Input: part model. Units: mm. Frame: model coordinates. A direction names the side the tool comes from. Give positions to 0.01 mm unless a question says otherwise; leave off trailing zeros. Write each loop counter-clockwise with the first axis right and the second up, starting at its lowest first coordinate (ties: lowest second). Pieces come first, ordered by that corner, then holes. Notation, with made-up numbers: (70, 74) -> (79, 74) arc R8 ccw to (79, 79) -> close; hole circle Ø9 at (-24, -7.5). An arc over 180 degrees is marked (long way). Return JSON: item names as keys, results as strings. Group by question number.
Item 1: Set-up query: faces 1 (the face through (143, 2, -49)), 2 (the face through (314.8, 0.99, -81.27)), 3 (the face through (163, 49, 0)), 4 (the face through (266.02, 0.99, -35.32)), 5 (the face through (143, 0, -51)). Return all of +Z, -Z, +X, -X, +Y, -Y with unobstructed straight access to the full face (end or side cutting, diameter ignored); none if empty.
Item 2: Section A-A, the plane y = 22. Return loops of the section in (x, z), then the cut area to 3 significant figures.
Item 3: Line query: line 1 (Z direction, x = 187, y = 1); line 2 (Z direction, x = -9, y = 61.5); line 3 (Y direction, x = 212.5, z = -59). Output: solid intervals per line, ascending. Write a range as [from, to].
Item 4: Pin query (flat end, axial travel): P1, Ø1.6, axis at y = 0.5, z = -47.5, coming from the +X side; P2, Ø5, axis at x = 196.5, y = 19, coming from the +Z side. Return the tip coordinate at first contact, or that it passes through.
Item 5: Mould query, pull axis X, two halves, no side actions, for faces 6 (the face through (266.84, 0.99, -66.93)), 7 (the face through (-50, 72.5, -98.4)), 8 (the face through (178, 98, -51)), 9 (the face through (340.31, 53.78, -0.99)). Classes: released by +X, released by -X, zero draft, split by the parting line, or undercut.
Item 6: Section D-D, the plane x = 93. Return loops of the section in (y, z), then the cut area to 3 significant figures.
Item 7: Section C-C, the plane z = -25. Return loops of the section in (x, y), then the cut area to 3 significant figures.
Item 8: Section B-B, the plane x = 151.5. Return loops of the section in (y, z).
Autodesk Inventor part; units mm, degrees
ref_plane "YZ Plane" through (0, 0, 0) normal (1, 0, 0) x (0, 1, 0)
ref_plane "XZ Plane" through (0, 0, 0) normal (0, 1, 0) x (-1, 0, 0)
ref_plane "XY Plane" through (0, 0, 0) normal (0, 0, 1) x (1, 0, 0)
sketch "Náčrt1" plane through (0, 0, 0) normal (1, 0, 0) x (0, 1, 0)
  line L0 (0, 0) -> (100, 0)
  line L1 (100, 0) -> (100, -100)
  line L2 (100, -100) -> (0, -100)
  line L3 (0, -100) -> (0, 0)
  line L4 (98, -2) -> (2, -2)
  line L5 (2, -2) -> (2, -98)
  line L6 (2, -98) -> (98, -98)
  line L7 (98, -98) -> (98, -2)
  dimension "d0" = 100
  dimension "d1" = 100
  dimension "d2" = 2
extrude "Vysunutí1" add sketch "Náčrt1" along normal blind 370
sketch "Náčrt4" plane through (0, 0, 0) normal (0, 0, 1) x (1, 0, 0)
  line L0 (0, 0) -> (0, 100)
  line L1 (0, 0) -> (370, 0)
  line L2 (370, 100) -> (370, 0)
  line L3 (0, 100) -> (370, 100)
  line L4 (0, 2) -> (370, 2)
  arc A0 (370, 98) -> (330.0148, 0) centre (465.2, 2) ccw
  line L5 (330, 23.5767) -> (330, -17.4459)
  line L6 (370, 2) -> (523.9799, 2)
  line L7 (330, 2) -> (370, 2)
  line L8 (0, 0) -> (370, 0)
  line L9 (370, 2) -> (370, 98)
  dimension "d17" = 2
  dimension "d102" = 330
extrude "Vysunutí4" cut sketch "Náčrt4" against normal through all contours A0 L2 L4 | L4 L2 L1 A0
sketch "Náčrt5" plane through (0, 100, 0) normal (0, 1, 0) x (1, 0, 0)
  line L0 (0, 0) -> (0, 100)
  line L1 (0, 0) -> (370, 0)
  line L2 (370, 100) -> (370, 0)
  line L3 (0, 100) -> (370, 100)
  arc A0 (370, 0) -> (370, 100) centre (343.3333, 50) ccw
  point P0 (400, 50)
  dimension "d21" = 30
extrude "Vysunutí5" add sketch "Náčrt5" against normal blind 2 contours L2 A0
sketch "Náčrt11" plane through (0, 0, -100) normal (0, -1, 0) x (1, 0, 0)
  line L0 (0, 100) -> (330.0148, 100)
  line L1 (0, 0) -> (0, 100)
  line L2 (0, 0) -> (330.0148, 0)
  line L3 (330.0148, 0) -> (330.0148, 100)
  line L4 (86.35, 55.65) -> (97.65, 55.65)
  line L5 (97.65, 55.65) -> (97.65, 44.35)
  line L6 (97.65, 44.35) -> (86.35, 44.35)
  line L7 (86.35, 44.35) -> (86.35, 55.65)
  point P0 (92, 55.65)
  point P1 (86.35, 50)
  dimension "d129" = 11.3
  dimension "d130" = 11.3
  dimension "d131" = 92
  dimension "d132" = 50
extrude "Vysunutí11" cut sketch "Náčrt11" against normal blind 5 contours L4 L5 L6 L7
sketch "Náčrt12" plane through (0, 0, -100) normal (0, -1, 0) x (1, 0, 0)
  line L0 (0, 100) -> (330.0148, 100)
  line L1 (0, 0) -> (0, 100)
  line L2 (0, 0) -> (330.0148, 0)
  circle A0 centre (187, 90) radius 2.25
  circle A1 centre (187, 10) radius 2.25
  line L3 (330.0148, 0) -> (330.0148, 100)
  dimension "d61" = 4.5
  dimension "d62" = 4.5
  dimension "d63" = 10
  dimension "d64" = 10
  dimension "d65" = 187
  dimension "d66" = 187
extrude "Vysunutí12" cut sketch "Náčrt12" against normal blind 10 contours A0 | A1
sketch "Náčrt14" plane through (0, 0, -100) normal (0, 0, -1) x (-1, 0, 0)
  line L0 (0, 0) -> (-330.0148, 0)
  line L1 (0, 100) -> (0, 0)
  line L2 (0, 100) -> (-370, 100)
  line L3 (-370, 98) -> (-370, 100)
  circle A0 centre (-293, 7.5) radius 2.25
  circle A1 centre (-293, 92.5) radius 2.25
  arc A2 (-330.0148, 0) -> (-370, 98) centre (-465.2, 2) ccw
  dimension "d77" = 293
  dimension "d78" = 4.5
  dimension "d79" = 4.5
  dimension "d80" = 293
  dimension "d86" = 85
  dimension "d87" = 7.5
extrude "Vysunutí14" cut sketch "Náčrt14" against normal through all contours A0 | A1
sketch "Náčrt16" plane through (0, 0, -100) normal (0, -1, 0) x (1, 0, 0)
  circle A0 centre (187, 90) radius 2.25
  circle A1 centre (187, 10) radius 2.25
  line L0 (330.0148, 0) -> (330.0148, 100)
  line L1 (0, 100) -> (330.0148, 100)
  line L2 (0, 0) -> (0, 100)
  line L3 (0, 0) -> (330.0148, 0)
  line L4 (0, 2) -> (330, 2)
  line L5 (0, 98) -> (330, 98)
  line L6 (300.0148, 65) -> (300.0148, 35)
  line L7 (300.0148, 35) -> (330, 2)
  line L8 (330, 2) -> (332.6841, 2)
  line L9 (332.6841, 2) -> (332.6841, 98)
  line L10 (332.6841, 98) -> (330, 98)
  line L11 (300.0148, 65) -> (330, 98)
  circle A2 centre (303.0148, 5) radius 2.5
  circle A3 centre (303.0148, 95) radius 2.5
  point P0 (300.0148, 50)
  dimension "d103" = 30
  dimension "d104" = 50
  dimension "d105" = 30
  dimension "d106" = 5
  dimension "d107" = 5
  dimension "d108" = 5
  dimension "d109" = 5
  dimension "d110" = 27
  dimension "d111" = 27
extrude "Vysunutí17" cut sketch "Náčrt16" against normal up to surface (2 mm away) contours L8 L7 L6 L11 L10 L0 | L0 L10 L9 L8 | A2 | A3
sketch "Náčrt17" plane through (0, 0, 0) normal (-1, 0, 0) x (0, 0, 1)
  line L0 (-98, 98) -> (-2, 98)
  line L1 (-2, 98) -> (-2, 2)
  line L2 (-2, 2) -> (-98, 2)
  line L3 (-98, 2) -> (-98, 98)
  line L4 (0, 0) -> (0, 100)
  line L5 (0, 100) -> (-100, 100)
  line L6 (-100, 100) -> (-100, 0)
  line L7 (-100, 0) -> (0, 0)
extrude "Vysunutí18" add sketch "Náčrt17" along normal blind 50
sketch "Náčrt18" plane through (-50, 100, 0) normal (0, 0, 1) x (1, 0, 0)
  arc A0 (420, -2) -> (380.0148, -100) centre (515.2, -98) ccw
  line L0 (420, 0) -> (420, -2)
  line L1 (420, 0) -> (0, 0)
  line L2 (0, -100) -> (0, 0)
  line L3 (0, -100) -> (380.0148, -100)
  circle A1 centre (5, -50) radius 1.75
  point P0 (50, -100)
  dimension "d116" = 3.5
  dimension "d117" = 50
  dimension "d118" = 5
extrude "Vysunutí19" cut sketch "Náčrt18" against normal through all contours A1
sketch "Náčrt19" plane through (300.0148, 0, -65) normal (0, -1, 0) x (1, 0, 0)
  line L0 (29.9852, 63) -> (30, 63)
  line L1 (30, 63) -> (30, 65)
  line L2 (-350.0148, 65) -> (30, 65)
  line L3 (-350.0148, -35) -> (-350.0148, 65)
  line L4 (30, -35) -> (-350.0148, -35)
  line L5 (30, -35) -> (30, -33)
  line L6 (30, -33) -> (29.9852, -33)
  line L7 (29.9852, -33) -> (0, 0)
  line L8 (0, 0) -> (0, 30)
  line L9 (0, 30) -> (29.9852, 63)
  circle A0 centre (3, 60) radius 2.5
  circle A1 centre (3, -30) radius 2.5
  circle A2 centre (-113.0148, 55) radius 2.25
  circle A3 centre (-113.0148, -25) radius 2.25
  circle A4 centre (-30, 29.5) radius 4
  circle A5 centre (-30, 0.5) radius 4
  point P0 (-300.0148, 65)
  dimension "d121" = 8
  dimension "d122" = 8
  dimension "d123" = 29
  dimension "d124" = 35.5
  dimension "d125" = 30
  dimension "d126" = 30
extrude "Vysunutí20" cut sketch "Náčrt19" against normal blind 10 contours A4 | A5
properties part number "Case"
Answer below:
{
 "1": {"face 1": "+X, -X", "face 2": "+X, -Y", "face 3": "+Z, +X, -X, +Y, -Y", "face 4": "-Y", "face 5": "+Z, -Z, +X, -X, -Y"},
 "2": {"outline": "(-50, -100) -> (331.49, -100) -> (331.49, -98) -> (-50, -98) -> close; (-50, -2) -> (331.49, -2) -> (331.49, 0) -> (-50, 0) -> close", "area": "1,530 mm2"},
 "3": {"line 1": "z = [-100, -92.25], [-87.75, -12.25], [-7.75, 0]", "line 2": "z = [-100, -98], [-2, 0]", "line 3": "y = [0, 2], [98, 100]"},
 "4": {"P1": "stops at x = 300.01", "P2": "stops at z = 0"},
 "5": {"face 6": "undercut", "face 7": "released by -X", "face 8": "zero draft", "face 9": "released by +X"},
 "6": {"outline": "(0, -100) -> (100, -100) -> (100, 0) -> (0, 0) -> (0, -44.35) -> (2, -44.35) -> (2, -2) -> (98, -2) -> (98, -98) -> (2, -98) -> (2, -55.65) -> (0, -55.65) -> close", "area": "761 mm2"},
 "7": {"outline": "(-50, 0) -> (309.1, 0) -> (309.1, 2) -> (-50, 2) -> close; (-50, 98) -> (394.19, 98) -> (394.19, 100) -> (-50, 100) -> close", "area": "1,610 mm2"},
 "8": {"outline": "(0, -100) -> (100, -100) -> (100, 0) -> (0, 0) -> close; hole (2, -98) -> (98, -98) -> (98, -2) -> (2, -2) -> close"}
}
